Input: part model. Units: mm. Frame: model coordinates. Face numbers are marked on the shaded views. A direction names the side the tool comes from. Coordinates: 2 decimals unless noted, no trailing zeros. Write each loop counter-clockwise with the first axis right and the second up, starting at its lowest first coordinate (ties: lowest second). Pieces come first, ordered by that corner, then holes.
1) Set-up query: the marked faces 1 and 2. Return all of +Z, -Z, +X, -X, +Y, -Y with unobstructed straight access to the full face (end or side cutting, diameter ignored); none if empty.
2) Section query A-A (z = 5.75). State how many separate pieces and enclosed holes the cut face has, then the cut area to 3 significant figures.
3) Pin query (flat end, axial travel): pin 1 Ø1.3 at (x, z) = (2, 6) entering from -Y; pin 2 Ø0.8 at (x, z) = (3, 6.5) entering from +Y; pin 3 Ø0.8 at (y, z) = (-5, 6) entering from +X. Return the tip coordinate at first contact, or that it passes through.
4) Line query: L1, parallel to Z at x = -21, y = 4; L2, parallel to X at y = 7, z = 6.25; L3, parallel to X at y = 5.5, z = 6.5. Output: solid intervals per line, ascending.
5) Section query B-B (x = 6). Output: boundary loops of the cut face in (y, z).
from build123d import *

# Parameters (mm, degrees)
F0_W     = 38.1
F0_H     = 38.1
F1_DEPTH = 5.08
F2_R     = 9.636419
F3_DEPTH = 2.54


with BuildPart() as f1:
    # F0 (on Top) → F1 (new body)
    with BuildSketch(Plane.XY):
        with Locations((-4.336205, -4.503883)):
            Rectangle(F0_W, F0_H)
    extrude(amount=F1_DEPTH)

    # F2 (on face) → F3 (join)
    with BuildSketch(Plane.XY.offset(5.08)):
        Polygon((-16.963584, 2.906272), (-16.933717, -11.906166), (-4.27773, -19.227108), (8.422415, -11.905848), (8.392711, 2.825718), (-4.27773, 10.219293), align=None)
        Polygon((-4.311768, -17.878222), (-15.968911, -11.225127), (-15.995917, 2.168256), (-4.333854, 8.891092), (7.299944, 2.28216), (7.327066, -11.168777), align=None, mode=Mode.SUBTRACT)
        Polygon((-15.133053, 1.699716), (-15.107919, -10.765341), (-4.311768, -17.065212), (6.484382, -10.841549), (6.484382, 1.714627), (-4.27773, 7.95749), align=None)
        with Locations((-4.31549, -4.503883)):
            Circle(F2_R, mode=Mode.SUBTRACT)
        with BuildLine():
            ThreePointArc((4.6324, -5.61813), (4.684216, -5.062077), (4.70151, -4.503883))
            ThreePointArc((4.70151, -4.503883), (4.687865, -4.008002), (4.646969, -3.513622))
            Line((4.646969, -3.513622), (0.866868, -3.513622))
            Line((0.866868, -3.513622), (4.410669, -2.232224))
            ThreePointArc((4.410669, -2.232224), (4.017353, -1.058594), (3.467016, 0.050114))
            Line((3.467016, 0.050114), (0.085442, -1.584476))
            Line((0.085442, -1.584476), (2.899253, 0.904792))
            ThreePointArc((2.899253, 0.904792), (2.101629, 1.830694), (1.186131, 2.640237))
            Line((1.186131, 2.640237), (-1.379733, -0.143722))
            Line((-1.379733, -0.143722), (0.269269, 3.26054))
            ThreePointArc((0.269269, 3.26054), (-0.836167, 3.814806), (-2.007042, 4.212616))
            Line((-2.007042, 4.212616), (-3.264274, 0.789716))
            Line((-3.264274, 0.789716), (-3.033893, 4.421574))
            ThreePointArc((-3.033893, 4.421574), (-4.351626, 4.513044), (-5.668584, 4.411016))
            Line((-5.668584, 4.411016), (-5.317712, 0.640375))
            Line((-5.317712, 0.640375), (-6.531781, 4.236502))
            ThreePointArc((-6.531781, 4.236502), (-7.775625, 3.822806), (-8.946344, 3.233137))
            Line((-8.946344, 3.233137), (-7.333815, -0.031659))
            Line((-7.333815, -0.031659), (-9.731831, 2.705106))
            ThreePointArc((-9.731831, 2.705106), (-10.684924, 1.878639), (-11.513346, 0.927245))
            Line((-11.513346, 0.927245), (-8.723363, -1.636518))
            Line((-8.723363, -1.636518), (-12.102514, 0.042383))
            ThreePointArc((-12.102514, 0.042383), (-12.655716, -1.076506), (-13.049107, -2.261068))
            Line((-13.049107, -2.261068), (-9.542109, -3.492343))
            Line((-9.542109, -3.492343), (-13.242584, -3.233735))
            ThreePointArc((-13.242584, -3.233735), (-13.33249, -4.504989), (-13.242272, -5.776221))
            Line((-13.242272, -5.776221), (-9.542109, -5.566502))
            Line((-9.542109, -5.566502), (-13.049957, -6.743385))
            ThreePointArc((-13.049957, -6.743385), (-12.648551, -7.948644), (-12.08175, -9.08553))
            Line((-12.08175, -9.08553), (-8.817994, -7.592915))
            Line((-8.817994, -7.592915), (-11.537476, -9.902884))
            ThreePointArc((-11.537476, -9.902884), (-10.695368, -10.875967), (-9.723315, -11.719264))
            Line((-9.723315, -11.719264), (-7.304202, -9.005236))
            Line((-7.304202, -9.005236), (-8.845366, -12.300454))
            ThreePointArc((-8.845366, -12.300454), (-7.737035, -12.846504), (-6.564463, -13.235917))
            Line((-6.564463, -13.235917), (-5.366502, -9.769401))
            Line((-5.366502, -9.769401), (-5.366502, -13.459421))
            ThreePointArc((-5.366502, -13.459421), (-4.208192, -13.520245), (-3.051657, -13.431874))
            Line((-3.051657, -13.431874), (-3.292344, -9.796692))
            Line((-3.292344, -9.796692), (-2.018305, -13.223358))
            ThreePointArc((-2.018305, -13.223358), (-0.859311, -12.832215), (0.23608, -12.287809))
            Line((0.23608, -12.287809), (-1.38217, -8.949596))
            Line((-1.38217, -8.949596), (1.108565, -11.707071))
            ThreePointArc((1.108565, -11.707071), (2.054256, -10.886095), (2.87708, -9.94201))
            Line((2.87708, -9.94201), (0.178137, -7.5158))
            Line((0.178137, -7.5158), (3.43137, -9.118257))
            ThreePointArc((3.43137, -9.118257), (4.000591, -7.989439), (4.406341, -6.792104))
            Line((4.406341, -6.792104), (0.937204, -5.61813))
            Line((0.937204, -5.61813), (4.6324, -5.61813))
        make_face()
    extrude(amount=F3_DEPTH)


solid = f1.part
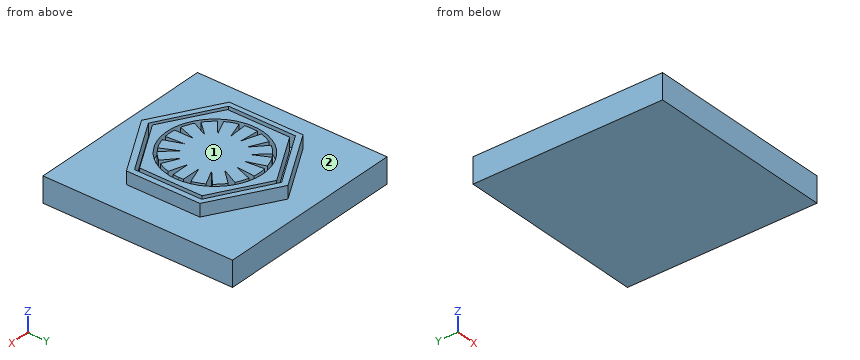
Answer:
1. face 1: +Z, +X, -X, +Y, -Y
1. face 2: +Z
2. separate pieces: 3
2. enclosed holes: 2
2. area: 431 mm2
3. pin 1: stops at y = -15.98
3. pin 2: stops at y = 6.21
3. pin 3: stops at x = 8.41
4. L1: z = 0 to 5.08
4. L2: x = -9.86 to -7.61, -5.94 to -2.63, -1 to 1.24
4. L3: x = -12.46 to -10.22, -8.54 to -0.04, 1.64 to 3.81
5. outline: (-23.55, 0) - (14.55, 0) - (14.55, 5.08) - (4.22, 5.08) - (4.22, 7.62) - (3.02, 7.62) - (3.02, 5.08) - (2, 5.08) - (2, 7.62) - (-11.12, 7.62) - (-11.12, 5.08) - (-11.93, 5.08) - (-11.93, 7.62) - (-13.3, 7.62) - (-13.3, 5.08) - (-23.55, 5.08) - close
